Autodesk Inventor part; units mm, degrees
ref_plane "YZ Plane" through (0, 0, 0) normal (1, 0, 0) x (0, 1, 0)
ref_plane "XZ Plane" through (0, 0, 0) normal (0, 1, 0) x (-1, 0, 0)
ref_plane "XY Plane" through (0, 0, 0) normal (0, 0, 1) x (1, 0, 0)
sketch "Эскиз1" plane through (0, 0, 0) normal (0, 1, 0) x (-1, 0, 0)
  line L0 (-13.3, -3.9495) -> (13.3, -3.9495)
  line L1 (13.3, -3.9495) -> (13.3, 3.9495)
  line L2 (13.3, 3.9495) -> (-13.3, 3.9495)
  line L3 (-13.3, 3.9495) -> (-13.3, -3.9495)
  line L4 (-13.3, -3.9495) -> (13.3, 3.9495) construction
  line L5 (13.3, -3.9495) -> (-13.3, 3.9495) construction
  line L6 (0, 3.9495) -> (0, -3.9495) construction
  circle A0 centre (0, 0.5505) radius 1.55
  circle A1 centre (-6.3, 0) radius 1.15
  circle A2 centre (9.7, 0) radius 1.15
  point P0 (0, 0)
  dimension "d0" = 13.3
  dimension "d1" = 7.899
  dimension "d2" = 3.1
  dimension "d3" = 4.5
  dimension "d35" = 2.3
  dimension "d36" = 2.3
  dimension "d37" = 7
  dimension "d38" = 16
  dimension "d39" = 3.9495
  dimension "d40" = 3.9495
extrude "Выдавливание1" add sketch "Эскиз1" along normal blind 4.5
sketch "Эскиз4" plane through (-13.3, 0, 3.9495) normal (0, 0, 1) x (1, 0, 0)
  line L0 (0, 0) -> (0, 4.5)
  line L1 (0, 0) -> (-8, 0)
  line L2 (0, 4.5) -> (26.6, 4.5)
  line L3 (-8, 0) -> (0, 4.5)
  point P0 (13.3, 0)
  point P1 (25.6, 4.5)
  point P2 (3.9103, 4.5)
  dimension "d19" = 8
extrude "Выдавливание4" add sketch "Эскиз4" against normal blind 7.899
fillet "Сопряжение4" radius 15 1 edges at (-13.3, 4.5, 0)
chamfer "Фаска2" distance 0.5 angle 45 1 edges at (1.55, 0, 0.5505)
chamfer "Фаска3" distance 1.1 angle 45 1 edges at (-4, 0, -3.9495)
fillet "Сопряжение7" radius 0.5 5 edges at (-4, 0, 3.9495) (-19.0123, 1.2868, 3.9495) (-13.1718, 4.0104, 3.9495) (1.9646, 4.5, 3.9495) (13.3, 4.5, 0)
chamfer "Фаска4" distance 1.5 angle 45 4 edges at (-8.55, 4.5, 0) (-10.4551, 4.4608, -0.8673) (-10.4603, 4.4604, 0.8628) (7.45, 4.5, 0)
equation "\"d39\" = 0.5 * d1"
equation "\"d40\" = d39"
properties part number "derz_LED"
Could you check a few things on this model? Use its own coordinates, in mm. A direction names the side the tool comes from. Coordinates: 2 decimals unless noted, no trailing zeros. Loops run counter-clockwise (first coordinate to the right, second up) from the corner with the lowest first, then second, coordinate; pieces in that order, holes last.
1) Will these pins go through, and if not, where does the flat tip stop? pin 1 Ø1 at (y, z) = (2.5, 1) entering from -X; pin 2 Ø1 at (y, z) = (3, 3) entering from -X; pin 3 Ø1.5 at (y, z) = (3.5, -1) entering from -X.
Reported:
pin 1: stops at x = -17.74
pin 2: stops at x = -16.86
pin 3: stops at x = -16.4
2) Which directions (+Z, -Z, +X, -X, +Y, -Y) give clear straight access to the entire face, cutting with the end or side of a thin tool? Please do faces 1 (the face through (-7.96, 3.59, 0.03)), 2 (the face through (-4, 0, 0)).
Reported:
face 1: +Y
face 2: +Z, -Z, +X, -X, -Y
3) Imagine slicing it at A-A (x = 6.3). List the corners of the cut face in (y, z) for me, and give its area (3 significant figures).
Reported:
outline: (0, -2.85) - (1.1, -3.95) - (4.5, -3.95) - (4.5, -2.65) - (3, -1.15) - (0, -1.15) - close; (0, 1.15) - (3, 1.15) - (4.5, 2.65) - (4.5, 3.45) arc R0.5 ccw to (4, 3.95) - (0.5, 3.95) arc R0.5 ccw to (0, 3.45) - close
area: 22.2 mm2
4) Please list where these lines run through material, in increasing order: line 1 along Z through (x, y) = (-9.7, 2.1); line 2 along Z through (x, y) = (0, 2.15); line 3 along X through (y, z) = (2.2, 0.5).
Reported:
line 1: z = -3.95 to -1.15, 1.15 to 3.95
line 2: z = -3.95 to -1, 2.1 to 3.95
line 3: x = -17.39 to -10.74, -8.66 to -1.55, 1.55 to 5.26, 7.34 to 13.3
5) Imagine slicing it at B-B (x = 11.5). List the corners of the cut face in (y, z) for me.
Reported:
outline: (0, -2.85) - (1.1, -3.95) - (4.5, -3.95) - (4.5, 3.45) arc R0.5 ccw to (4, 3.95) - (0.5, 3.95) arc R0.5 ccw to (0, 3.45) - close
